Build history of the part. All positions in model axes, mm. A direction names the side the tool comes from. Round coordinates to 2 decimals unless told otherwise and drop trailing zeros. Loops run counter-clockwise (first coordinate to the right, second up) from the corner with the lowest first, then second, coordinate; pieces in that order, holes last. Notation, with made-up numbers: (16.25, 20.25) - (25.25, 20.25) arc R30 ccw to (25.25, 59.25) - close; hole circle Ø8 at (-19, -19.75). An arc over 180 degrees is marked (long way). Use one line per item in the form item = value. Start each with the question number.
Q1. Mould opens along Z. For faces 1 (the face through (-12.25, 2.21, 1.95)), 2 (the face through (12.5, 2, 5)), 3 (the face through (0, 9, 10)) say: released by +Z, released by -Z, zero draft, split by the parting line, or undercut.
Q2. Drill centre lines: line 1 (Z direction, x = 11, y = 2.3); line 2 (X direction, y = 0.7, z = 8); line 3 (Y direction, x = 10.75, z = 5.75). Where is each one in solid material? Low to high.
Q3. Saw through at B-B (x = 11). Give the cut face in (y, z), then the cut area to 3 significant figures.
Q4. 3-axis set-ups, long thin cutter, end or side, ignore diameter. For faces 4 (the face through (11.8, 0.7, 2.6)), 5 (the face through (10.01, 2.21, 8.76)), 6 (the face through (0, 9, 0)), 7 (the face through (-11, 3, 5)), 8 (the face through (11, 3, 5)): which of +Z, -Z, +X, -X, +Y, -Y reach the whole face in a straight line?
Q5. Pin check, flat tips, straight feed: pin 1 (3 mm diameter, centred on x = 10.5, z = 8, fed in from +Y); pin 2 (1.5 mm diameter, centred on x = 11, z = 6, fed in from +Y); pin 3 (1.5 mm diameter, centred on x = 2.5, z = 8.5, fed in from +Y). Stop position of each tip, or through.
Q6. Saw through at D-D (z = 6.25). Give the cut face in (x, y), then the cut area to 3 significant figures.
Q7. Saw through at C-C (y = 7). Give the cut face in (x, z), then the cut area to 3 significant figures.
Q8. Saw through at A-A (z = 8). Give the cut face in (x, y), then the cut area to 3 significant figures.
```python
from build123d import *

# Parameters (mm, degrees)
SALIENTE_EXTRUIR1_DEPTH                              = 10
REFRENTADO_PARA_TORNILLO_CON_CABEZA_TRON_D           = 2
REFRENTADO_PARA_TORNILLO_CON_CABEZA_TRON_CBORE_D     = 2.5
REFRENTADO_PARA_TORNILLO_CON_CABEZA_TRON_CBORE_DEPTH = 1.6


with BuildPart() as part:
    # Croquis1 → Saliente-Extruir1 (new body)
    with BuildSketch(Plane.XY):
        with BuildLine():
            ThreePointArc((-9.5, 3), (0, 9.962429423), (9.5, 3))
            Line((9.5, 3), (12.5, 3))
            Line((12.5, 3), (12.5, 0))
            Line((12.5, 0), (8.5, 0))
            ThreePointArc((8.5, 0), (0, 8.5), (-8.5, 0))
            Line((-8.5, 0), (-12.5, 0))
            Line((-12.5, 0), (-12.5, 3))
            Line((-12.5, 3), (-9.5, 3))
        make_face()
    extrude(amount=SALIENTE_EXTRUIR1_DEPTH)

    # Refrentado para tornillo con cabeza troncocónica de M23 (through all)
    with Locations(Plane(origin=(-11, 3, 2), x_dir=(1, 0, 0), z_dir=(0, 1, 0))):
        with Locations((0, 0), (0, -6), (22, 0), (22, -6)):
            CounterBoreHole(REFRENTADO_PARA_TORNILLO_CON_CABEZA_TRON_D / 2, REFRENTADO_PARA_TORNILLO_CON_CABEZA_TRON_CBORE_D / 2, REFRENTADO_PARA_TORNILLO_CON_CABEZA_TRON_CBORE_DEPTH)


solid = part.part
```
Report:
q1.face_1 = undercut
q1.face_2 = zero draft
q1.face_3 = released by +Z
q2.line_1 = 0 to 0.75, 3.25 to 6.75, 9.25 to 10
q2.line_2 = -12.5 to -12, -10 to -8.47, 8.47 to 10, 12 to 12.5
q2.line_3 = 0 to 3
q3.outline = (0, 0) - (3, 0) - (3, 0.75) - (1.4, 0.75) - (1.4, 1) - (0, 1) - close; (0, 3) - (1.4, 3) - (1.4, 3.25) - (3, 3.25) - (3, 6.75) - (1.4, 6.75) - (1.4, 7) - (0, 7) - close; (0, 9) - (1.4, 9) - (1.4, 9.25) - (3, 9.25) - (3, 10) - (0, 10) - close
q3.area = 16.4 mm²
q4.face_4 = +Y, -Y
q4.face_5 = +Y
q4.face_6 = -Z, +X, -X, +Y, -Y
q4.face_7 = +Z, -Z, -X, +Y
q4.face_8 = +Z, -Z, +X, +Y
q5.pin_1 = 4.27
q5.pin_2 = 3
q5.pin_3 = 9.81
q6.outline = (-12.5, 0) - (-8.5, 0) arc R8.5 cw to (8.5, 0) - (12.5, 0) - (12.5, 3) - (9.5, 3) arc R9.96 ccw to (-9.5, 3) - (-12.5, 3) - close
q6.area = 58.6 mm²
q7.outline = (-7.09, 0) - (-4.82, 0) - (-4.82, 10) - (-7.09, 10) - close; (4.82, 0) - (7.09, 0) - (7.09, 10) - (4.82, 10) - close
q7.area = 45.3 mm²
q8.outline = (-12.5, 0) - (-12, 0) - (-12, 1.4) - (-12.25, 1.4) - (-12.25, 3) - (-12.5, 3) - close; (-10, 0) - (-8.5, 0) arc R8.5 cw to (8.5, 0) - (10, 0) - (10, 1.4) - (9.75, 1.4) - (9.75, 3) - (9.5, 3) arc R9.96 ccw to (-9.5, 3) - (-9.75, 3) - (-9.75, 1.4) - (-10, 1.4) - close; (12, 0) - (12.5, 0) - (12.5, 3) - (12.25, 3) - (12.25, 1.4) - (12, 1.4) - close
q8.area = 45.0 mm²
